Can you work these out from the model? Positions are in its coordinate system, mm. Face numbers are marked on the shaded views. A direction names the side the tool comes from. Coordinates: 2 decimals unless noted, no trailing zeros. Order: outer loops, then holes, each group sorted by start corner. A loop starts at its lowest first (then second) coordinate and runs counter-clockwise, first axis right, second up. Notation, with made-up numbers: (74.5, 19.25) -> (132.5, 19.25) arc R21 ccw to (132.5, 56.25) -> close; hole circle Ø8 at (35.5, 78). An arc over 180 degrees is marked (long way). Use a Markdown table: item, result. Add a question column.
1. Suppose I cut it at D-D, the plane y = 29. List the corners of the cut face in (x, z) for me, then the cut area to 3 significant figures.
2. We'd pull the mould along Z, two halves only. Please class the marked faces 1, 2 and 3: pulls with the +Z half, pulls with the -Z half, needs draft (parallel to the pull), parting line crosses it, or undercut.
3. If I drill on line 1 along Z through (x, y) = (0, -21); line 2 along X through (y, z) = (4, 25); line 3 along Z through (x, y) = (-32, -7), over which ranges is the centre line in solid material (lowest first)? Write a range as from..to.
4. For the marked faces 4 and 5, which set-ups out of +Z, -Z, +X, -X, +Y, -Y let a thin tool reach every point of the face, with its end or its side?
5. For pin 1 Ø1 at (x, z) = (-53, 52) entering from +Y; pin 2 Ø8 at (x, z) = (-5, 57.5) entering from -Y; pin 3 Ø2 at (x, y) = (-20, 10) entering from +Z; pin 4 Ø5 at (y, z) = (-13, 58) entering from -X, each with a flat end and sliding along its axis, tell me the tip position at first contact or that it passes through.
6. Suppose I cut it at C-C, the plane x = -50.8. List the corners of the cut face in (y, z) for me (3 decimals).
7. Suppose I cut it at A-A, the plane x = 0. List the corners of the cut face in (y, z) for me (3 decimals).
8. Suppose I cut it at B-B, the plane z = 25.4. List the corners of the cut face in (x, y) for me (3 decimals).
```python
from build123d import *

# Parameters (mm, degrees)
F0_W     = 152.4
F0_H     = 69.85
F1_DEPTH = 50.8
F2_R     = 19.05
F3_DEPTH = 201.422
F4_R     = 6.35
F5_DEPTH = 25.4


with BuildPart() as f1:
    # F0 (on Top) → F1 (new body)
    with BuildSketch(Plane.XY):
        Rectangle(F0_W, F0_H)
    extrude(amount=F1_DEPTH)

    # F2 (on face) → F3 (cut)
    with BuildSketch(Plane.XZ.offset(34.925)):
        with Locations((0, 25.4)):
            Circle(F2_R)
    extrude(amount=-F3_DEPTH, mode=Mode.SUBTRACT)

    # F4 (on face) → F5 (join)
    with BuildSketch(Plane.XY.offset(50.8)):
        with Locations((50.8, 9.525)):
            Circle(F4_R)
        with Locations((-50.8, -9.525)):
            Circle(F4_R)
    extrude(amount=F5_DEPTH)


solid = f1.part
```
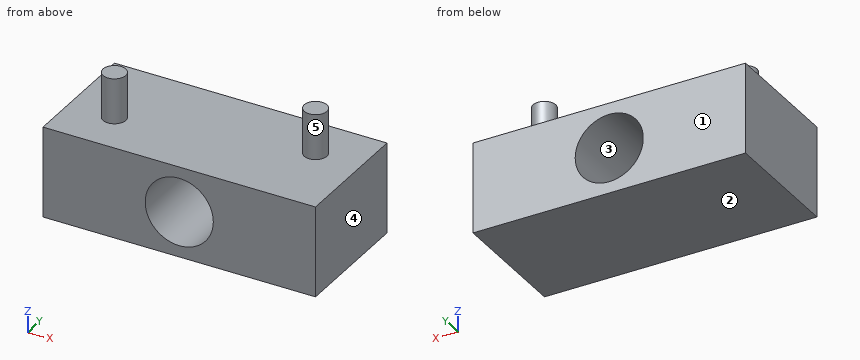
Worked out:
| question | item | result |
|---|---|---|
| 1 | outline | (-76.2, 0) -> (76.2, 0) -> (76.2, 50.8) -> (-76.2, 50.8) -> close; hole circle Ø38.1 at (0, 25.4) |
| 1 | area | 6,600 mm² |
| 2 | face 1 | needs draft |
| 2 | face 2 | pulls with the -Z half |
| 2 | face 3 | undercut |
| 3 | line 1 | z = 0..6.35, 44.45..50.8 |
| 3 | line 2 | x = -76.2..-19.05, 19.05..76.2 |
| 3 | line 3 | z = 0..50.8 |
| 4 | face 4 | +Z, -Z, +X, +Y, -Y |
| 4 | face 5 | +Z |
| 5 | pin 1 | stops at y = -3.41 |
| 5 | pin 2 | passes through |
| 5 | pin 3 | stops at z = 50.8 |
| 5 | pin 4 | stops at x = -57.07 |
| 6 | outline | (-34.925, 0) -> (34.925, 0) -> (34.925, 50.8) -> (-3.175, 50.8) -> (-3.175, 76.2) -> (-15.875, 76.2) -> (-15.875, 50.8) -> (-34.925, 50.8) -> close |
| 7 | outline | (-34.925, 0) -> (34.925, 0) -> (34.925, 6.35) -> (-34.925, 6.35) -> close; (-34.925, 44.45) -> (34.925, 44.45) -> (34.925, 50.8) -> (-34.925, 50.8) -> close |
| 8 | outline | (-76.2, -34.925) -> (-19.05, -34.925) -> (-19.05, 34.925) -> (-76.2, 34.925) -> close; (19.05, -34.925) -> (76.2, -34.925) -> (76.2, 34.925) -> (19.05, 34.925) -> close |
